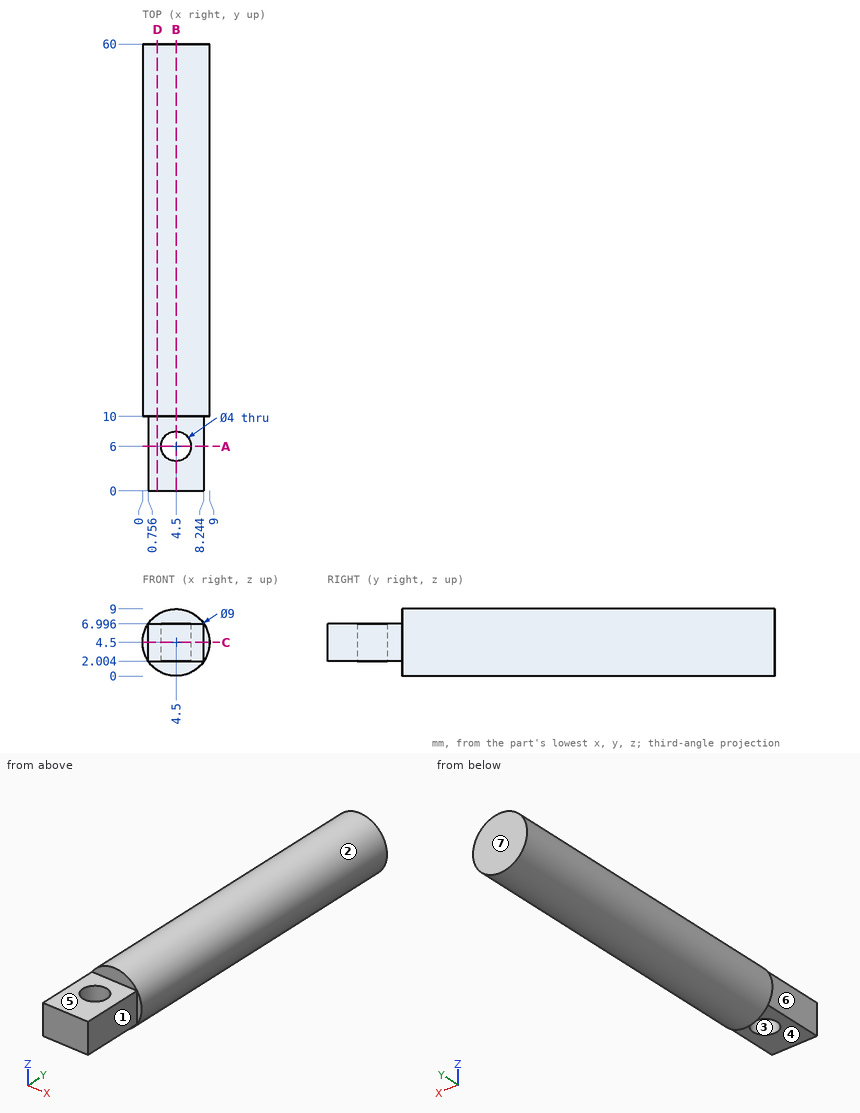
For this review, use the dimensioned drawing (mm, ordinates from the lowest corner) and the shaded views. A direction names the side the tool comes from. Round coordinates to 2 decimals unless told otherwise and drop trailing zeros. Order: outer loops, then holes, each group sorted by start corner. A loop starts at its lowest first (then second) coordinate and runs counter-clockwise, first axis right, second up. Notation, with made-up numbers: M 20.5,7.5 L 50.5,7.5 A32 cw 50.5,35.5 Z; hole C 67.5,-16 d9. An arc over 180 degrees is marked long. Use a Markdown table: item, result.
1) Consider section B-B (x = 4.5). Write out the cut boundary in (y, z), then the cut area to 3 significant figures.
Report:
| item | result |
|---|---|
| outline | M 0,2 L 4,2 L 4,7 L 0,7 Z; M 8,2 L 10,2 L 10,0 L 60,0 L 60,9 L 10,9 L 10,7 L 8,7 Z |
| area | 480 mm^2 |
2) Wall thickness on line 1 along Y through (x, z) = (4.5, 4.35); line 2 along Z through (x, y) = (7, 31); line 3 along Z through (x, y) = (5.75, 8): over which ranges is each line inside the solid? List them lowest first. Write a range as [from, to].
Report:
| item | result |
|---|---|
| line 1 | [0, 4], [8, 60] |
| line 2 | [0.76, 8.24] |
| line 3 | [2, 7] |
3) Consider section A-A (y = 6). Write out the cut boundary in (x, z).
Report:
| item | result |
|---|---|
| outline | M 0.76,2 L 2.5,2 L 2.5,7 L 0.76,7 Z; M 6.5,2 L 8.24,2 L 8.24,7 L 6.5,7 Z |
4) Tool access review of the marked faces 5, 6 and 7: name each direction out of +Z, -Z, +X, -X, +Y, -Y from which nothing blocks a thin tool from reaching the whole face with its end or side.
Report:
| item | result |
|---|---|
| face 5 | +Z, +X, -X, -Y |
| face 6 | +Z, -Z, -X, -Y |
| face 7 | +Z, -Z, +X, -X, +Y |
5) Draft analysis for pull direction X (two halves, no side actions). For the marked faces 1, 2, 3 and 4, state which applies: released by +X, released by -X, zero draft, split by the parting line, or undercut.
Report:
| item | result |
|---|---|
| face 1 | released by +X |
| face 2 | split by the parting line |
| face 3 | undercut |
| face 4 | zero draft |
6) Insertion check: pin 1 (4.5 mm diameter, centred on x = 4.5, y = 6, fed in from -Z); pin 2 (2.5 mm diameter, centred on y = 6.5, z = 5, fed in from -X); pin 3 (2 mm diameter, centred on y = 51, z = 8, fed in from +X). Each pin has a flat end and moves straight along its axis. Give the tip position at first contact, or say it passes through.
Report:
| item | result |
|---|---|
| pin 1 | z = 2 |
| pin 2 | x = 0.76 |
| pin 3 | x = 8.24 |
7) Consider section D-D (x = 2). Write out the cut boundary in (y, z).
Report:
| item | result |
|---|---|
| outline | M 0,2 L 10,2 L 10,0.76 L 60,0.76 L 60,8.24 L 10,8.24 L 10,7 L 0,7 Z |
8) Consider section C-C (z = 4.5). Write out the cut boundary in (x, y), then the cut area to 3 significant figures.
Report:
| item | result |
|---|---|
| outline | M 0,10 L 0.76,10 L 0.76,0 L 8.24,0 L 8.24,10 L 9,10 L 9,60 L 0,60 Z; hole C 4.5,6 d4 |
| area | 512 mm^2 |
